from build123d import *

# Parameters (mm, degrees)
F0_W      = 100
F0_H      = 20
F1_DEPTH  = 27.5
F2_W      = 190
F2_H      = 30
F3_DEPTH  = 55.001
F4_W      = 30
F4_H      = 45
F5_DEPTH  = 500
F6_R      = 2.5
F7_DEPTH  = 40.001
F8_R      = 2.5
F9_DEPTH  = 60.001
F10_R     = 2.5
F11_DEPTH = 60.001
F12_W     = 145.98173
F12_H     = 84.634348
F12_W_2   = 100
F12_H_2   = 25
F13_DEPTH = 20


with BuildPart() as f1:
    # F0 (on Top) → F1 (new body, symmetric)
    with BuildSketch(Plane.XY):
        Polygon((100, 0), (-100, 0), (-100, -40), (-50, -40), (50, -40), (100, -40), align=None)
        with Locations((0, -50)):
            Rectangle(F0_W, F0_H)
    extrude(amount=F1_DEPTH, both=True)

    # F2 (on face) → F3 (cut, through all)
    with BuildSketch(Plane.XY.offset(27.5)):
        with Locations((0, -20)):
            Rectangle(F2_W, F2_H)
    extrude(amount=-F3_DEPTH, mode=Mode.SUBTRACT)

    # F4 (on face) → F5 (cut, symmetric)
    with BuildSketch(Plane.YZ.offset(-95)):
        with Locations((-20, 0)):
            Rectangle(F4_W, F4_H)
    extrude(amount=F5_DEPTH, both=True, mode=Mode.SUBTRACT)

    # F6 (on face) → F7 (cut, through all)
    with BuildSketch(Plane.XZ.offset(40)):
        with Locations((-90, 0)):
            Circle(F6_R)
        with Locations((90, 0)):
            Circle(F6_R)
    extrude(amount=-F7_DEPTH, mode=Mode.SUBTRACT)

    # F8 (on face) → F9 (cut, through all)
    with BuildSketch(Plane.XZ.offset(60)):
        with Locations((-45, 0)):
            Circle(F8_R)
        with Locations((45, 0)):
            Circle(F8_R)
    extrude(amount=-F9_DEPTH, mode=Mode.SUBTRACT)

    # F10 (on face) → F11 (cut, through all)
    with BuildSketch(Plane.XZ.offset(60)):
        Circle(F10_R)
    extrude(amount=-F11_DEPTH, mode=Mode.SUBTRACT)

    # F12 (on face) → F13 (cut, through all)
    with BuildSketch(Plane.XZ.offset(60)):
        Rectangle(F12_W, F12_H)
        Rectangle(F12_W_2, F12_H_2, mode=Mode.SUBTRACT)
    extrude(amount=-F13_DEPTH, mode=Mode.SUBTRACT)


solid = f1.part
Verification items for the finished model (mm, model axes). A direction names the side the tool comes from. Give positions to 0.01 mm unless a question says otherwise; leave off trailing zeros. Order: outer loops, then holes, each group sorted by start corner. A loop starts at its lowest first (then second) coordinate and runs counter-clockwise, first axis right, second up. Notation, with made-up numbers: M -5,12.5 L 28,12.5 A14 ccw 28,16.5 Z; hole C 11,-7.75 d1. An arc over 180 degrees is marked long. Answer as a JSON object with one key per item and string values. Group by question number.
1) Access from +Z, -Z, +X, -X, +Y, -Y to the whole of each face (thin tool, end or side, straight path). Record for faces 4 (the face through (50, -50, 0)), 5 (the face through (95, -20, 25)), 6 (the face through (-97, -20, -22.5)), 7 (the face through (-50, -50, 0)).
2) Cross-section at B-B (y = -25). Enter the section's corners in (x, z).
3) Cross-section at C-C (x = 90). Enter the section's corners in (y, z), then the cut area to 3 significant figures.
4) Scan lines: line 1 along Y through (x, z) = (81.5, -3.5); line 2 along X through (y, z) = (-28.5, 23); line 3 along Y through (x, z) = (10.5, -7). Record each from-to range of solid material in increasing order. Write a range as [from, to].
5) Cross-section at A-A (x = 36). Enter the section's corners in (y, z), then the cut area to 3 significant figures.
6) Depth check by flat-ended pin: pin 1 Ø1.5 at (x, y) = (-33, -48.5) entering from +Z; pin 2 Ø4 at (x, z) = (20, 18.5) entering from -Y; pin 3 Ø10 at (y, z) = (-54, -3) entering from +X. Enter the tip coordinate at first touch or a pass-through.
7) Mould release check, pull along Y, two halves, no side actions. Record for faces 1 (the face through (98, -20, -22.5)), 2 (the face through (98, -20, 22.5)), 3 (the face through (87.5, -37.5, 0.1)): released by +Y, released by -Y, zero draft, split by the parting line, or undercut.
8) Cross-section at D-D (z = -16.5). Enter the section's corners in (x, y).
Result sheet:
{
 "1": {"face 4": "+Z, -Z, +X, -Y", "face 5": "+Z, -Z", "face 6": "+X, -X", "face 7": "+Z, -Z, -X, -Y"},
 "2": {"outline": "M -100,-27.5 L -95,-27.5 L -95,-22.5 L -100,-22.5 Z; M -100,22.5 L -95,22.5 L -95,27.5 L -100,27.5 Z; M 95,-27.5 L 100,-27.5 L 100,-22.5 L 95,-22.5 Z; M 95,22.5 L 100,22.5 L 100,27.5 L 95,27.5 Z"},
 "3": {"outline": "M -40,-27.5 L -35,-27.5 L -35,-2.5 L -40,-2.5 Z; M -40,2.5 L -35,2.5 L -35,27.5 L -40,27.5 Z; M -5,-27.5 L 0,-27.5 L 0,-2.5 L -5,-2.5 Z; M -5,2.5 L 0,2.5 L 0,27.5 L -5,27.5 Z", "area": "500 mm2"},
 "4": {"line 1": "y = [-40, -35], [-5, 0]", "line 2": "x = [-100, -95], [95, 100]", "line 3": "y = [-60, -35], [-5, 0]"},
 "5": {"outline": "M -60,-12.5 L -40,-12.5 L -40,-27.5 L -35,-27.5 L -35,27.5 L -40,27.5 L -40,12.5 L -60,12.5 Z; M -5,-27.5 L 0,-27.5 L 0,27.5 L -5,27.5 Z", "area": "1,050 mm2"},
 "6": {"pin 1": "stops at z = 12.5", "pin 2": "stops at y = -40", "pin 3": "stops at x = 50"},
 "7": {"face 1": "undercut", "face 2": "undercut", "face 3": "zero draft"},
 "8": {"outline": "M -100,-40 L 100,-40 L 100,-35 L -100,-35 Z; M -100,-5 L 100,-5 L 100,0 L -100,0 Z"}
}
